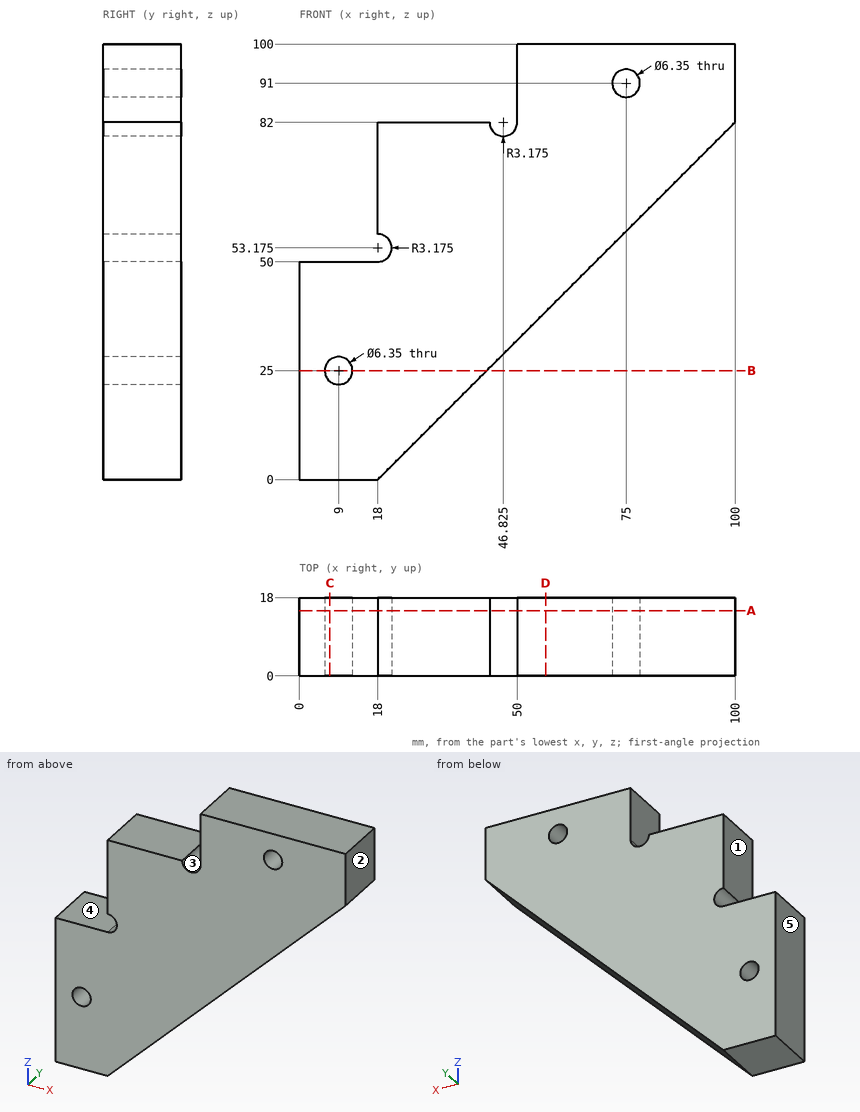
Check sheet for the drawn part. Datum: minimum x, y, z corner. Units: mm. A direction names the side the tool comes from. Round coordinates to 2 decimals unless told otherwise and drop trailing zeros. Order: outer loops, then holes, each group sorted by start corner. A loop starts at its lowest first (then second) coordinate and runs counter-clockwise, first axis right, second up.
1. Section check D-D on x = 56.5. Record the cut outline in (y, z).
Final values:
outline: (0, 38.5) - (18, 38.5) - (18, 100) - (0, 100) - close
2. Thickness scan on L1, parallel to X at y = 9, z = 91 (3 decimals); L2, parallel to Z at x = 9, y = 7.5 (3 decimals); L3, parallel to Z at x = 75, y = 12.5 (3 decimals). Record the ranges inside material, lowest first.
Final values:
L1: x = 50 to 71.825, 78.175 to 100
L2: z = 0 to 21.825, 28.175 to 50
L3: z = 57 to 87.825, 94.175 to 100
3. Release check for a two-part mould opening along X. For the marked faces 3, 4 and 5 record: +X half, -X half, draft (parallel to the pull), parting line (faces both ways), or undercut.
Final values:
face 3: undercut
face 4: draft
face 5: -X half
4. Section check A-A on y = 15. Record the cut outline in (x, z) (3 decimals), then the cut area to 3 significant figures.
Final values:
outline: (0, 0) - (18, 0) - (100, 82) - (100, 100) - (50, 100) - (50, 82) arc R3.175 cw to (43.65, 82) - (18, 82) - (18, 56.35) arc R3.175 cw to (18, 50) - (0, 50) - close; hole circle Ø6.35 at (9, 25); hole circle Ø6.35 at (75, 91)
area: 5,070 mm2
5. Go/stop test with flat-tipped pins: P1, Ø6, axis at x = 82, y = 11.5, coming from the -Z side; P2, Ø8, axis at y = 10.5, z = 15, coming from the +X side; P3, Ø1.5, axis at y = 14.5, z = 63.5, coming from the +X side. Record where each tip stops, or that it passes through.
Final values:
P1: stops at z = 61
P2: stops at x = 37
P3: stops at x = 82.25
6. Section check C-C on x = 7. Record the cut outline in (y, z).
Final values:
outline: (0, 0) - (18, 0) - (18, 22.53) - (0, 22.53) - close; (0, 27.47) - (18, 27.47) - (18, 50) - (0, 50) - close
7. Access from +Z, -Z, +X, -X, +Y, -Y to the whole of each face (thin tool, end or side, straight path). Record for the marked faces 1 and 2.
Final values:
face 1: +Z, -X, +Y, -Y
face 2: +Z, -Z, +X, +Y, -Y
8. Section check B-B on z = 25. Record the cut outline in (x, y) (3 decimals), then the cut area to 3 significant figures.
Final values:
outline: (0, 0) - (5.825, 0) - (5.825, 18) - (0, 18) - close; (12.175, 0) - (43, 0) - (43, 18) - (12.175, 18) - close
area: 660 mm2
